```python
from build123d import *

# Parameters (mm, degrees)
F1_DEPTH = 1000


with BuildPart() as f1:
    # F0 (on Front) → F1 (new body)
    with BuildSketch(Plane.XZ):
        with BuildLine():
            Line((-15, 0), (0, 0))
            Line((0, 0), (15, 0))
            Line((15, 0), (15, 5))
            Line((15, 5), (3, 5))
            Line((3, 5), (3, 8.803848))
            ThreePointArc((3, 8.803848), (5.795555, 15.552914), (0, 20))
            ThreePointArc((0, 20), (-5.795555, 15.552914), (-3, 8.803848))
            Line((-3, 8.803848), (-3, 5))
            Line((-3, 5), (-15, 5))
            Line((-15, 5), (-15, 0))
        make_face()
    extrude(amount=F1_DEPTH)


solid = f1.part
```
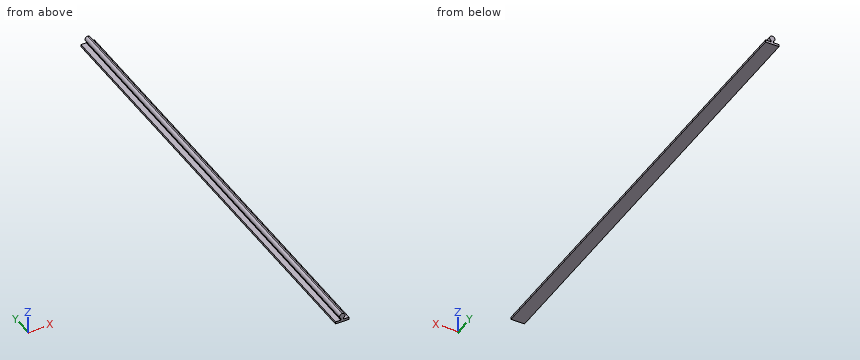
Read the model definition and answer for the solid it produces. Units are mm, in the model's axes. Coordinates: 2 decimals unless noted, no trailing zeros. Loops run counter-clockwise (first coordinate to the right, second up) from the corner with the lowest first, then second, coordinate; pieces in that order, holes last. Notation, with made-up numbers: (-24.5, -38) - (27.5, -38) arc R30 ccw to (27.5, 1) - close; hole circle Ø1 at (75, 87). An arc over 180 degrees is marked (long way). Answer in a Markdown table with one row per item.
1. Given pin 1 (1.1 mm diameter, centred on y = -575.5, z = 6.5, fed in from -X); pin 2 (10 mm diameter, centred on y = -457, z = 12, fed in from -X); pin 3 (3.5 mm diameter, centred on x = -8.5, y = -353.5, fed in from +Z), each flat-ended and moving along its own axis, determine where each tip first touches the part or whether it passes through.
Conclusion:
| item | result |
|---|---|
| pin 1 | stops at x = -3 |
| pin 2 | stops at x = -6 |
| pin 3 | stops at z = 5 |
2. Find section A-A, the plane y = -901.5. Write down the section's boundary in (x, z).
Conclusion:
| item | result |
|---|---|
| outline | (-15, 0) - (15, 0) - (15, 5) - (3, 5) - (3, 8.8) arc R6 ccw (long way) to (-3, 8.8) - (-3, 5) - (-15, 5) - close |
3. Straight lines are drawn through the part: line 1 (Z direction, x = 13.75, y = -700.5); line 2 (Z direction, x = 0.5, y = -336); line 3 (X direction, y = -731.5, z = 8.5). For each, find the intervals that lie inside material, in ascending order.
Conclusion:
| item | result |
|---|---|
| line 1 | z = 0 to 5 |
| line 2 | z = 0 to 19.98 |
| line 3 | x = -3 to 3 |
4. Find section B-B, the plane z = 12. Write down the section's boundary in (x, y).
Conclusion:
| item | result |
|---|---|
| outline | (-5.66, -1000) - (5.66, -1000) - (5.66, 0) - (-5.66, 0) - close |
